Verification items for the finished model (mm, model axes). A direction names the side the tool comes from. Coordinates: 2 decimals unless noted, no trailing zeros. Write each loop counter-clockwise with the first axis right and the second up, starting at its lowest first coordinate (ties: lowest second). Pieces come first, ordered by that corner, then holes. Notation, with made-up numbers: M 71.25,-20.75 L 108.25,-20.75 A30 cw 108.25,18.25 Z; hole C -14.5,15 d1. An arc over 180 degrees is marked long. One line per item, written item: value.
```python
from build123d import *

# Parameters (mm, degrees)
SKETCH_2_W          = 40
SKETCH_2_H          = 40
EXTRUDE_2_DEPTH     = 1
SKETCH_3_R          = 2
CUT_EXTRUDE_2_DEPTH = 10
SKETCH_2_10_W       = 19.5
SKETCH_2_10_H       = 19.5
CUT_EXTRUDE_3_DEPTH = 10


with BuildPart() as part:
    # Sketch 2 → Extrude 2 (new body)
    with BuildSketch(Plane(origin=(0, 0, 0), x_dir=(1, 0, 0), z_dir=(0, 1, 0))):
        Rectangle(SKETCH_2_W, SKETCH_2_H)
    extrude(amount=EXTRUDE_2_DEPTH)

    # Sketch 3 → Cut-Extrude 2 (cut)
    with BuildSketch(Plane(origin=(0, 0, 0), x_dir=(1, 0, 0), z_dir=(0, 1, 0))):
        with Locations(Location((-15.224798987, -15.224798987, 0), (0, 0, 270))):
            Circle(SKETCH_3_R)
        with Locations(Location((15.224798987, -15.224798987, 0), (0, 0, 270))):
            Circle(SKETCH_3_R)
        with Locations(Location((15.224798987, 15.224798987, 0), (0, 0, 270))):
            Circle(SKETCH_3_R)
        with Locations(Location((-15.224798987, 15.224798987, 0), (0, 0, 270))):
            Circle(SKETCH_3_R)
    extrude(amount=CUT_EXTRUDE_2_DEPTH, mode=Mode.SUBTRACT)

    # Sketch 2_10 → Cut-Extrude 3 (cut)
    with BuildSketch(Plane(origin=(0, 0, 0), x_dir=(1, 0, 0), z_dir=(0, 1, 0))):
        Rectangle(SKETCH_2_10_W, SKETCH_2_10_H)
    extrude(amount=CUT_EXTRUDE_3_DEPTH, mode=Mode.SUBTRACT)


solid = part.part
```
Item 1: Draft check along X on faces 1 (the face through (0, 1, -14)), 2 (the face through (-9.75, 0.5, 0.1)), 3 (the face through (-20, 0.5, 0.3)). Enter one of: released by +X, released by -X, zero draft, split by the parting line, or undercut.
The answers:
face 1: zero draft
face 2: undercut
face 3: released by -X
Item 2: Cross-section at C-C, the plane y = 0.4. Enter the section's corners in (x, z).
The answers:
outline: M -20,-20 L 20,-20 L 20,20 L -20,20 Z; hole C -15.22,-15.22 d4; hole C -15.22,15.22 d4; hole M -9.75,-9.75 L 9.75,-9.75 L 9.75,9.75 L -9.75,9.75 Z; hole C 15.22,-15.22 d4; hole C 15.22,15.22 d4
Item 3: Cross-section at D-D, the plane z = -15.5. Enter the section's corners in (x, y).
The answers:
outline: M -20,0 L -17.21,0 L -17.21,1 L -20,1 Z; M -13.24,0 L 13.24,0 L 13.24,1 L -13.24,1 Z; M 17.21,0 L 20,0 L 20,1 L 17.21,1 Z
Item 4: Go/stop test with a flat-tipped pin: P1, Ø4.5, axis at x = -15.22, z = -15.22, coming from the -Y side. Record where the tip stops, or that it passes through.
The answers:
P1: stops at y = 0
Item 5: Cross-section at A-A, the plane z = -1.5. Enter the section's corners in (x, y), and give its area (3 significant figures).
The answers:
outline: M -20,0 L -9.75,0 L -9.75,1 L -20,1 Z; M 9.75,0 L 20,0 L 20,1 L 9.75,1 Z
area: 20.5 mm²
Item 6: Access from +Z, -Z, +X, -X, +Y, -Y to the whole of each face (thin tool, end or side, straight path). Record for faces 4 (the face through (-0.1, 0.5, -9.75)), 5 (the face through (20, 0.5, 0.3)).
The answers:
face 4: +Y, -Y
face 5: +Z, -Z, +X, +Y, -Y
Item 7: Scan lines: line 1 (Z direction, x = 3.5, y = 0.6); line 2 (X direction, y = 0.35, z = -16). Record each from-to range of solid material in increasing order.
The answers:
line 1: z = -20 to -9.75, 9.75 to 20
line 2: x = -20 to -17.07, -13.38 to 13.38, 17.07 to 20
Item 8: Cross-section at B-B, the plane x = 0. Enter the section's corners in (y, z).
The answers:
outline: M 0,-20 L 1,-20 L 1,-9.75 L 0,-9.75 Z; M 0,9.75 L 1,9.75 L 1,20 L 0,20 Z
